Autodesk Inventor part; units mm, degrees
ref_plane "YZ Plane" through (0, 0, 0) normal (1, 0, 0) x (0, 1, 0)
ref_plane "XZ Plane" through (0, 0, 0) normal (0, 1, 0) x (-1, 0, 0)
ref_plane "XY Plane" through (0, 0, 0) normal (0, 0, 1) x (1, 0, 0)
sketch "Sketch1" plane through (0, 0, 0) normal (0, 0, 1) x (1, 0, 0)
  line L0 (0, 0) -> (19.05, 0)
  line L1 (19.05, 0) -> (19.05, -2.3622)
  line L2 (19.05, -2.3622) -> (14.8082, -2.3622)
  line L3 (14.8082, -2.3622) -> (14.8082, -8.7122)
  line L4 (14.8082, -8.7122) -> (0, -8.7122)
  line L5 (0, -8.7122) -> (0, 0)
  dimension "d2" = 19.05
  dimension "d3" = 2.3622
  dimension "d4" = 4.2418
  dimension "d5" = 6.35
revolve "Revolution1" add sketch "Sketch1" angle 360 about axis through (0, -8.7122, 0) along (0, 1, 0)
sketch "Sketch2" plane through (0, 0, 0) normal (0, 1, 0) x (1, 0, 0)
  circle A0 centre (0, 0) radius 12.7
  dimension "d7" = 25.4
extrude "Extrusion1" cut sketch "Sketch2" against normal blind 25.4
sketch "Sketch3" plane through (0, -8.7122, 0) normal (0, -1, 0) x (1, 0, 0)
  circle A0 centre (0, 0) radius 14.2875
  circle A1 centre (0, 0) radius 14.8082
  dimension "d10" = 28.575
extrude "Extrusion2" cut sketch "Sketch3" against normal blind 6.35
properties part number "BevelWheelSpace_Clearance" material "ABS Plastic"
Input: part model. Units: mm. Frame: model coordinates. A direction names the side the tool comes from. Give positions to 0.01 mm unless a question says otherwise; leave off trailing zeros. Order: outer loops, then holes, each group sorted by start corner. A loop starts at its lowest first (then second) coordinate and runs counter-clockwise, first axis right, second up.
Q1. Contact query for flat-ended pins moving along their axis: pin 1 Ø5 at (x, y) = (-6.5, -6.5) entering from +Z; pin 2 Ø4 at (x, y) = (-3, -5) entering from -Z; pin 3 Ø2 at (x, y) = (10.5, -1.5) entering from -Z. Output: stop coordinate, or through.
Checked values:
pin 1: stops at z = 13.72
pin 2: stops at z = -14.25
pin 3: stops at z = -16.51
Q2. Section B-B on z = 6.5. Output: boundary loops of the cut face in (x, y).
Checked values:
outline: (-17.91, -2.36) - (-12.72, -2.36) - (-12.72, -8.71) - (-10.91, -8.71) - (-10.91, 0) - (-17.91, 0) - close; (10.91, -8.71) - (12.72, -8.71) - (12.72, -2.36) - (17.91, -2.36) - (17.91, 0) - (10.91, 0) - close
Q3. Set-up query: faces 1 (the flat face through (-13, -8.712, 1)), 2 (the flat face through (2.7, -2.362, -14.2)). Return all of +Z, -Z, +X, -X, +Y, -Y with unobstructed straight access to the full face (end or side cutting, diameter ignored); none if empty.
Checked values:
face 1: +Z, -Z, +X, -X, -Y
face 2: -Y
Q4. Section D-D on y = -7. Output: boundary loops of the cut face in (x, z) (1 decimal), and give its area (3 significant figures).
Checked values:
outline: circle Ø28.6 at (0, 0); hole circle Ø25.4 at (0, 0)
area: 135 mm2
Q5. Section C-C on y = -1. Output: boundary loops of the cut face in (x, z).
Checked values:
outline: circle Ø38.1 at (0, 0); hole circle Ø25.4 at (0, 0)
Q6. Ray query, probe 1 along Z at (x, y) = (0, -1.75); probe 2 along Z at (x, y) = (0, -6). Return the intervals inside material, ascending.
Checked values:
probe 1: z = -19.05 to -12.7, 12.7 to 19.05
probe 2: z = -14.29 to -12.7, 12.7 to 14.29
Q7. Section A-A on x = 0. Output: boundary loops of the cut face in (y, z), and give its area (3 significant figures).
Checked values:
outline: (-8.71, -14.29) - (-2.36, -14.29) - (-2.36, -19.05) - (0, -19.05) - (0, -12.7) - (-8.71, -12.7) - close; (-8.71, 12.7) - (0, 12.7) - (0, 19.05) - (-2.36, 19.05) - (-2.36, 14.29) - (-8.71, 14.29) - close
area: 50.2 mm2
Q8. Draft query along X for faces 3 (the cylindrical face through (-2.75, -4.3, 12.4)), 4 (the flat face through (12.4, 0, 4)), 5 (the cylindrical face through (-15.12, -1.2, -11.59)). Return one class per face: +X half, -X half, draft (parallel to the pull), parting line (faces both ways), or undercut.
Checked values:
face 3: undercut
face 4: draft
face 5: parting line
